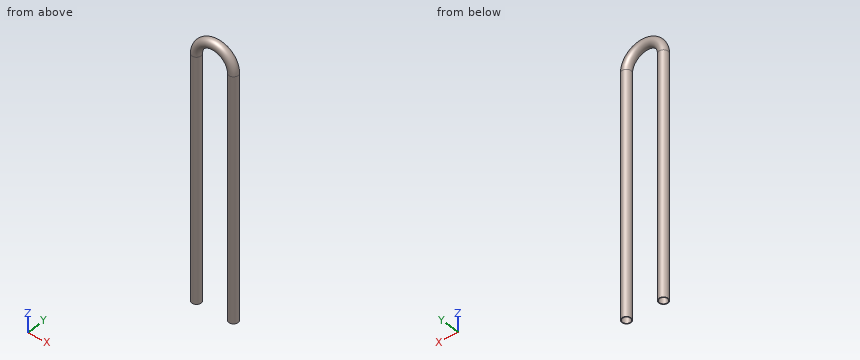
Solid Edge part; units mm, degrees
sketch "Sketch1" plane through (0, 0, 0) normal (0, -1, 0) x (1, 0, 0)
  line L0 (0, 0) -> (0, 655)
sketch "Sketch2" plane through (0, 0, 0) normal (0, 0, -1) x (-1, 0, 0)
  circle A0 centre (0, 0) radius 12.5
sweep "SweptProtrusion_8" add profiles "Sketch2" path "Sketch1"
sketch "Sketch3" plane through (0, 0, 0) normal (0, -1, 0) x (1, 0, 0)
  arc A0 (0, 655) -> (100, 655) centre (50, 655) cw
sketch "Sketch4" plane through (0, 0, 655) normal (0, 0, 1) x (-1, 0, 0)
  circle A0 centre (0, 0) radius 12.5
sweep "SweptProtrusion_10" add profiles "Sketch4" path "Sketch3"
sketch "Sketch5" plane through (0, 0, 0) normal (0, -1, 0) x (1, 0, 0)
  line L0 (100, 655) -> (100, 0)
sketch "Sketch6" plane through (100, 0, 655) normal (0, 0, -1) x (0, 1, 0)
  circle A0 centre (0, 0) radius 12.5
sweep "SweptProtrusion_11" add profiles "Sketch6" path "Sketch5"
shell "Thinwall_2" thickness 2 removed faces 4 at (8.5833, -8.0833, 0) at (108.5833, -8.0833, 0) at (8.5833, -8.0833, 0) at (108.5833, -8.0833, 0)
properties material "Stainless steel"
The model under review builds one solid part; all positions refer to its coordinate system, in mm. Round coordinates to 2 decimals unless told otherwise and drop trailing zeros. Write each loop counter-clockwise with the first axis right and the second up, starting at its lowest first coordinate (ties: lowest second). Pieces come first, ordered by that corner, then holes. Notation, with made-up numbers: (79.5, -38.75) - (100.5, -38.75) arc R16 cw to (100.5, -30.75) - close; hole circle Ø1 at (53, -15). An arc over 180 degrees is marked (long way). Answer as CSV lines item,"result". Start each with the question number.
(1) We need section A-A on y = 0. State the section outline as (x, z) points, plus the area to 3 significant figures.
(2) For pin 1 Ø2 at (x, z) = (94.5, 510.5) entering from +Y; pin 2 Ø8 at (x, z) = (92.5, 491.5) entering from +Y; pin 3 Ø2 at (y, z) = (-2.5, 344) entering from -X, all flat-tipped, find the tip position at first contact; note any pin that passes through.
(3) To check wall thickness, follow line 1 (X direction, y = 1, z = 221.5); line 2 (X direction, y = -6, z = 408); line 3 (Y direction, x = 100, z = 137). State the ranges of each line that lie inside material, in increasing order.
(4) We need section B-B on z = 612. State the section outline as (x, y) points.
Worked answers:
1,outline,"(-12.5, 0) - (-10.5, 0) - (-10.5, 655) arc R60.5 cw to (110.5, 655) - (110.5, 0) - (112.5, 0) - (112.5, 655) arc R62.5 ccw to (-12.5, 655) - close; (10.5, 0) - (12.5, 0) - (12.5, 655) arc R37.5 cw to (87.5, 655) - (87.5, 0) - (89.5, 0) - (89.5, 655) arc R39.5 ccw to (10.5, 655) - close"
1,area,"5,870 mm²"
2,pin 1,"y = 11.66"
2,pin 2,"y = 12"
2,pin 3,"x = -12.41"
3,line 1,"-12.46 to -10.45, 10.45 to 12.46, 87.54 to 89.55, 110.45 to 112.46"
3,line 2,"-10.97 to -8.62, 8.62 to 10.97, 89.03 to 91.38, 108.62 to 110.97"
3,line 3,"-12.5 to -10.5, 10.5 to 12.5"
4,outline,"circle Ø25 at (0, 0); circle Ø25 at (100, 0); hole circle Ø21 at (0, 0); hole circle Ø21 at (100, 0)"
